Input: part model. Units: mm. Frame: model coordinates. A direction names the side the tool comes from. Round coordinates to 2 decimals unless told otherwise and drop trailing zeros. Write each loop counter-clockwise with the first axis right and the second up, starting at its lowest first coordinate (ties: lowest second). Pieces come first, ordered by that corner, then holes. Notation, with made-up numbers: (-38, 18.25) -> (-18, 18.25) arc R18 ccw to (-18, 25.25) -> close; hole circle Ø7 at (26, 10). An arc over 180 degrees is marked (long way). Write item = value, one per line.
Autodesk Inventor part; units mm, degrees
ref_plane "YZ Plane" through (0, 0, 0) normal (1, 0, 0) x (0, 1, 0)
ref_plane "XZ Plane" through (0, 0, 0) normal (0, 1, 0) x (-1, 0, 0)
ref_plane "XY Plane" through (0, 0, 0) normal (0, 0, 1) x (1, 0, 0)
sketch "Sketch1" plane through (0, 0, 0) normal (0, 1, 0) x (-1, 0, 0)
  line L0 (4.7625, -2.7496) -> (0, -5.4993)
  line L1 (0, -5.4993) -> (-4.7625, -2.7496)
  line L2 (-4.7625, -2.7496) -> (-4.7625, 2.7496)
  line L3 (-4.7625, 2.7496) -> (0, 5.4993)
  line L4 (0, 5.4993) -> (4.7625, 2.7496)
  line L5 (4.7625, 2.7496) -> (4.7625, -2.7496)
  point P0 (0, 0)
  point P1 (0, 0)
  dimension "d0" = 9.525
extrude "Extrusion1" add sketch "Sketch1" along normal blind 5.1562
sketch "Sketch2" plane through (0, 5.1562, 0) normal (0, 1, 0) x (1, 0, 0)
  circle A0 centre (0, 0) radius 2.413
  dimension "d3" = 4.826
extrude "Extrusion2" add sketch "Sketch2" along normal blind 25.4
properties part number "10-32 bolt"
1) Line query: L1, parallel to Y at x = 2.25, z = -3.25; L2, parallel to X at y = 29.5, z = 0; L3, parallel to Z at x = 0.5, y = 24. Output: solid intervals per line, ascending. Write a range as from..to.
Solutions:
L1 = 0..5.16
L2 = -2.41..2.41
L3 = -2.36..2.36
2) Cut plane C-C (x = -1). Return the cut outline in (y, z).
Solutions:
outline = (0, -4.92) -> (5.16, -4.92) -> (5.16, -2.2) -> (30.56, -2.2) -> (30.56, 2.2) -> (5.16, 2.2) -> (5.16, 4.92) -> (0, 4.92) -> close
3) Cut plane D-D (x = 3.75). Return the cut outline in (y, z), and give its area (3 significant figures).
Solutions:
outline = (0, -3.33) -> (5.16, -3.33) -> (5.16, 3.33) -> (0, 3.33) -> close
area = 34.4 mm^2
4) Cut plane B-B (y = 27). Return the cut outline in (x, z), and give its area (3 significant figures).
Solutions:
outline = circle Ø4.83 at (0, 0)
area = 18.3 mm^2
5) Cut plane A-A (z = 0). Return the cut outline in (x, y).
Solutions:
outline = (-4.76, 0) -> (4.76, 0) -> (4.76, 5.16) -> (2.41, 5.16) -> (2.41, 30.56) -> (-2.41, 30.56) -> (-2.41, 5.16) -> (-4.76, 5.16) -> close
6) First-contact query: P1, Ø2, axis at y = 9, z = -2, coming from the -X side; P2, Ø6, axis at y = 16.5, z = -4, coming from the +X side; P3, Ø3, axis at x = -2, y = 21.5, coming from the -Z side. Flat tips, straight axial feed; report the tip coordinate or a pass-through.
Solutions:
P1 = -2.2
P2 = 2.2
P3 = -2.36
7) Access query for faces 1 (the face through (1.1, 5.156, -2.4)), 2 (the face through (4.762, 3, 0)). Directions: +Z, -Z, +X, -X, +Y, -Y. A direction counts if a zero-diameter tool reaches every point of the face in a straight line with its end or side. Return the directions, or none.
Solutions:
face_1 = +Y
face_2 = +Z, -Z, +X, +Y, -Y
